from build123d import *

# Parameters (mm, degrees)
F1_W     = 30
F1_H     = 30
F1_R     = 1.75
F2_DEPTH = 3
F0_W     = 30
F0_H     = 30
F0_R     = 1.75
F3_DEPTH = 3
F5_W     = 30
F5_H     = 30
F5_R     = 1.75
F6_DEPTH = 3
F7_R     = 1


# Not quite as in the source:
# - a fillet or chamfer that OpenCascade refuses, or shapes differently, is made with other operations: its cross-section is extruded or revolved along the edge and cut away or added


with BuildPart() as f2:
    # F1 (on Right) → F2 (new body)
    with BuildSketch(Plane.YZ):
        with Locations((15, 15)):
            Rectangle(F1_W, F1_H)
        with Locations((15, 15)):
            Circle(F1_R, mode=Mode.SUBTRACT)
    extrude(amount=F2_DEPTH)

    # F0 (on Top) → F3 (join)
    with BuildSketch(Plane.XY):
        with Locations((15, 15)):
            Rectangle(F0_W, F0_H)
        with Locations((15, 15)):
            Circle(F0_R, mode=Mode.SUBTRACT)
    extrude(amount=F3_DEPTH)

    # F5 (on face) → F6 (join)
    with BuildSketch(Plane.XZ.offset(-30)):
        with Locations((15, 15)):
            Rectangle(F5_W, F5_H)
        with Locations((15, 15)):
            Circle(F5_R, mode=Mode.SUBTRACT)
    extrude(amount=F6_DEPTH)

    # F7
    f7_edges = [f2.edges().sort_by_distance(p)[0] for p in [
        (3, 13.5, 3),
        (3, 13.5, 30),
        (30, 13.5, 3),
        (3, 0, 16.5),
        (16.5, 0, 3),
        (16.5, 27, 3),
        (16.5, 27, 30),
        (3, 27, 16.5),
        (30, 27, 16.5),
    ]]
    fillet(f7_edges, radius=F7_R)

    # F8: fillet of radius 4 on 1 edges, made by hand

    # F8_s1 → F8_t2 (revolve, cut)
    with BuildSketch(Plane.XZ.offset(-15)):
        with BuildLine():
            ThreePointArc((16.75, 0), (18.1734936034, 2.1622776602), (20.6229833462, 3))
            Line((20.6229833462, 3), (16.75, 3))
            Line((16.75, 3), (16.75, 0))
        make_face()
    revolve(axis=Axis((15, 15, 3), (0, 0, 1)), mode=Mode.SUBTRACT)

    # F9: fillet of radius 4 on 1 edges, made by hand

    # F9_s1 → F9_t2 (revolve, cut)
    with BuildSketch(Plane.XY.offset(15)):
        with BuildLine():
            ThreePointArc((3, 20.6229833462), (2.1622776602, 18.1734936034), (0, 16.75))
            Line((0, 16.75), (3, 16.75))
            Line((3, 16.75), (3, 20.6229833462))
        make_face()
    revolve(axis=Axis((3, 15, 15), (1, 0, 0)), mode=Mode.SUBTRACT)

    # F10: fillet of radius 3.5 on 1 edges, made by hand

    # F10_s1 → F10_t2 (revolve, cut)
    with BuildSketch(Plane.XY.offset(15)):
        with BuildLine():
            ThreePointArc((20.2141016151, 27), (17.9228137677, 27.8542486889), (16.75, 30))
            Line((16.75, 30), (16.75, 27))
            Line((16.75, 27), (20.2141016151, 27))
        make_face()
    revolve(axis=Axis((15, 27, 15), (0, -1, 0)), mode=Mode.SUBTRACT)


solid = f2.part
Verification items for the finished model (mm, model axes). A direction names the side the tool comes from. Coordinates: 2 decimals unless noted, no trailing zeros. Loops run counter-clockwise (first coordinate to the right, second up) from the corner with the lowest first, then second, coordinate; pieces in that order, holes last. Notation, with made-up numbers: (-38, 19) -> (-1, 19) arc R30 cw to (-1, 49) -> close; hole circle Ø8 at (33.5, 23). An arc over 180 degrees is marked (long way). Answer as a JSON object with one key per item and string values. Group by question number.
Item 1: Scan lines: probe 1 along Y at (x, z) = (28.75, 7); probe 2 along X at (y, z) = (20.25, 26). Record each from-to range of solid material in increasing order.
Item 2: Sectioned sample at C-C on y = 14. State how many separate pieces and enclosed holes the cut face has, plus the area to 3 significant figures.
Item 3: Depth check by flat-ended pin: pin 1 (4 mm diameter, centred on x = 16.5, z = 21, fed in from -Y); pin 2 (3 mm diameter, centred on y = 17.5, z = 12.5, fed in from +X). Enter the tip coordinate at first touch or a pass-through.
Item 4: Tool access check on faces 1 (the cylindrical face through (17.182, 27.301, 29.715)), 2 (the flat face through (15, 30, 11)). Record the directions out of +Z, -Z, +X, -X, +Y, -Y that give a thin tool (end or side, any length) a straight path to the whole face; none if there is none.
Item 5: Sectioned sample at A-A on x = 5.75. Record the boundary of the cut face in (y, z), plus the area to 3 significant figures.
Item 6: Sectioned sample at B-B on z = 8.75. Record the boundary of the cut face in (x, y), plus the area to 3 significant figures.
Evaluation:
{
 "1": {"probe 1": "y = 27 to 30", "probe 2": "x = 0 to 3"},
 "2": {"separate pieces": "3", "enclosed holes": "0", "area": "140 mm²"},
 "3": {"pin 1": "stops at y = 27", "pin 2": "stops at x = 2.96"},
 "4": {"face 1": "+Z, +X, -Y", "face 2": "+Z, -Z, +X, -X, +Y"},
 "5": {"outline": "(0, 0) -> (30, 0) -> (30, 30) -> (28, 30) arc R1 ccw to (27, 29) -> (27, 4) arc R1 cw to (26, 3) -> (1, 3) arc R1 ccw to (0, 2) -> close", "area": "171 mm²"},
 "6": {"outline": "(0, 0) -> (2, 0) arc R1 ccw to (3, 1) -> (3, 26) arc R1 cw to (4, 27) -> (29, 27) arc R1 ccw to (30, 28) -> (30, 30) -> (0, 30) -> close", "area": "171 mm²"}
}
